Part model, mm, in its own coordinate system. A direction names the side the tool comes from. Round coordinates to 2 decimals unless told otherwise and drop trailing zeros. Loops run counter-clockwise (first coordinate to the right, second up) from the corner with the lowest first, then second, coordinate; pieces in that order, holes last. Notation, with made-up numbers: M 12,5.25 L 31,5.25 A15 ccw 31,15.25 Z; hole C -32.5,66.25 d10. An arc over 180 degrees is marked long. Put each result on its own line as item: value. Start each with the question number.
1) Slice it at B-B on x = 0. Give the cut face in (y, z).
2) Which spindle directions (+Z, -Z, +X, -X, +Y, -Y) get a long thin tool onto all of the face, cutting with end or side? Do faces 1 (the cylindrical face through (10.79, -23.59, -21.2)), 2 (the flat face through (-6.35, -13, -99)). Say none if no direction does.
3) Slice it at D-D on x = 9.5. Give the cut face in (y, z), then the cut area to 3 significant figures.
4) Probe line 1 along Z through (x, y) = (0, -4.75); line 2 along Z through (x, y) = (-0.75, -18.25); line 3 along X through (y, z) = (-14, 52.5). List the from-to ranges inside material, lowest first.
5) Pull direction X, two halves, no side cores. Call faces 3 (the flat face through (12.7, -13, -24)), 4 (the cylindrical face through (-10.89, -23.49, -21.2)), 5 (the flat face through (0, -13, -105.67)): +X half, -X half, draft (parallel to the pull), parting line (faces both ways), or undercut.
6) Drop flat-ended pins along their axis: pin 1 Ø1.5 at (x, z) = (-9.5, -8) entering from -Y; pin 2 Ø1.5 at (y, z) = (-4.5, -51.5) entering from +X. Give the stop position or say it passes through.
7) Slice it at C-C on y = -10.5. Give the cut face in (x, z).
```python
from build123d import *

# Parameters (mm, degrees)
F1_DEPTH = 25.4
F3_D     = 12.7
F3_DEPTH = 254
F3_TIP   = 3.8154649308
F4_W     = 25.4
F4_H     = 82.55
F5_DEPTH = 25.4
F7_DEPTH = 25.4
F8_R     = 6.34999


# Not quite as in the source:
# - a fillet or chamfer is up to 0.001 mm smaller than in the source, because OpenCascade refuses the exact size


with BuildPart() as f1:
    # F0 (on Front) → F1 (new body)
    with BuildSketch(Plane.XZ):
        Polygon((-12.7, -32.0098340811), (0, -32.0098340811), (12.7, -32.0098340811), (12.7, 69.5901659189), (-12.7, 69.5901659189), align=None)
    extrude(amount=F1_DEPTH)

    # F3
    with Locations(Plane.XZ.offset(25.4)):
        with Locations((0, 56.8901659189)):
            Hole(F3_D / 2, depth=F3_DEPTH)
            with Locations((0, 0, -(F3_DEPTH + F3_TIP / 2))):  # 118° drill point
                Cone(0, F3_D / 2, F3_TIP, mode=Mode.SUBTRACT)

    # F4 (on face) → F5 (join)
    with BuildSketch(Plane.XZ.offset(25.4)):
        with Locations((0, -73.2848340811)):
            Rectangle(F4_W, F4_H)
    extrude(amount=-F5_DEPTH)

    # F6 (on face) → F7 (cut)
    with BuildSketch(Plane(origin=(0, 0, 0), x_dir=(-1, 0, 0), z_dir=(0, 1, 0))):
        Polygon((0, -105.6698340811), (6.35, -105.6698340811), (6.35, -92.9698340811), (-6.35, -92.9698340811), (-6.35, -105.6698340811), align=None)
    extrude(amount=-F7_DEPTH, mode=Mode.SUBTRACT)

    # F8 (radius 6.35 in the source; OpenCascade refuses exactly that, so slightly less here)
    f8_edges = [f1.edges().sort_by_distance(p)[0] for p in [
        (12.7, 0, -22.484834),
        (-12.7, 0, -22.484834),
        (-12.7, -25.4, -22.484834),
        (12.7, -25.4, -22.484834),
    ]]
    fillet(f8_edges, radius=F8_R)


solid = f1.part
```
Recorded:
1. outline: M -25.4,-114.56 L 0,-114.56 L 0,-105.67 L -25.4,-105.67 Z; M -25.4,-92.97 L 0,-92.97 L 0,50.54 L -25.4,50.54 Z; M -25.4,63.24 L 0,63.24 L 0,69.59 L -25.4,69.59 Z
2. face 1: +Z, -Z, +X, -Y
2. face 2: +Y, -Y
3. outline: M -24.56,-114.56 L -0.84,-114.56 L -0.84,69.59 L -24.56,69.59 Z
3. area: 4,370 mm2
4. line 1: z = -114.56 to -105.67, -92.97 to 50.54, 63.24 to 69.59
4. line 2: z = -114.56 to -105.67, -92.97 to 50.58, 63.2 to 69.59
4. line 3: x = -12.7 to -4.59, 4.59 to 12.7
5. face 3: +X half
5. face 4: -X half
5. face 5: undercut
6. pin 1: stops at y = -24.93
6. pin 2: stops at x = 12.6
7. outline: M -12.7,-114.56 L 12.7,-114.56 L 12.7,69.59 L -12.7,69.59 Z; hole M -6.35,-105.67 L 6.35,-105.67 L 6.35,-92.97 L -6.35,-92.97 Z; hole C 0,56.89 d12.7
